Source: CAD feature listing. Evaluate the final solid. Frame: model axes, mm. A direction names the side the tool comes from. Give positions to 0.01 mm unless a question says otherwise; leave off trailing zeros. Order: outer loops, then holes, each group sorted by start corner. A loop starts at its lowest first (then second) coordinate and runs counter-clockwise, first axis right, second up.
1) First-contact query: P1, Ø8.5, axis at y = 16, z = -265.5, coming from the +X side; P2, Ø3, axis at x = -2, z = -152.5, coming from the +Y side; P3, Ø4, axis at y = 10, z = -219, coming from the -X side. Flat tips, straight axial feed; report the tip coordinate or a pass-through.
2) Access query for faces 1 (the face through (-9, 25, 0)), 2 (the face through (-5.622, 33, -211)), 3 (the face through (-9, 25, -428.625)), 4 (the face through (-6.511, 32, -211)), 5 (the face through (-2.967, 3.174, -211.312)). Directions: +Z, -Z, +X, -X, +Y, -Y. A direction counts if a zero-diameter tool reaches every point of the face in a straight line with its end or side. Return the directions, or none.
3) Draft query along Y for faces 6 (the face through (-10.739, 42.804, -211.312)), 7 (the face through (-8.767, 16, -211)), 8 (the face through (-3.45, 2.413, -211.312)), 9 (the face through (-9.656, 16, -211)). Return one class per face: released by +Y, released by -Y, zero draft, split by the parting line, or undercut.
4) Section A-A, the plane x = -2.25. Return loops of the section in (y, z) (3 decimals), plus the area to 3 significant figures.
5) Section C-C, the plane y = 15. Return loops of the section in (x, z) (3 decimals), plus the area to 3 significant figures.
6) Material intervals for line 1 (X direction, y = 32.5, z = -94); line 2 (X direction, y = 29, z = -211.5); line 3 (X direction, y = 20, z = -220.5), sorted ascending.
```python
from build123d import *

# Parameters (mm, degrees)
EXTRUDE_THIN1_DEPTH = 428.625
FILLET1_R           = 0.889


with BuildPart() as part:
    # Sketch1 → Extrude-Thin1 (new body)
    with BuildSketch(Plane.XY):
        with BuildLine():
            ThreePointArc((0, 0), (4.964730566, 2.465229927), (7.9375, 7.14375))
            Line((7.9375, 7.14375), (11.1125, 7.14375))
            Line((11.1125, 7.14375), (11.1125, 24.60625))
            ThreePointArc((11.1125, 24.60625), (12.04243597, 26.85131403), (14.2875, 27.78125))
            Line((14.2875, 27.78125), (13.517722525, 32.146875))
            Line((13.517722525, 32.146875), (16.898645987, 34.098852071))
            ThreePointArc((16.898645987, 34.098852071), (18.624416275, 36.126706761), (18.680023291, 38.788921177))
            ThreePointArc((18.680023291, 38.788921177), (12.079369103, 42.78588283), (7.078269835, 36.909375))
            Line((7.078269835, 36.909375), (7.078269835, 28.178125))
            Line((7.078269835, 28.178125), (0.728269835, 28.178125))
            Line((0.728269835, 28.178125), (0.728269835, 27.289125))
            Line((0.728269835, 27.289125), (7.967269835, 27.289125))
            Line((7.967269835, 27.289125), (7.967269835, 36.909375))
            ThreePointArc((7.967269835, 36.909375), (12.221538279, 41.908324327), (17.836494775, 38.508242281))
            ThreePointArc((17.836494775, 38.508242281), (17.79334373, 36.442363895), (16.454145987, 34.868748655))
            Line((16.454145987, 34.868748655), (12.534135133, 32.605529333))
            Line((12.534135133, 32.605529333), (13.251696834, 28.536034702))
            ThreePointArc((13.251696834, 28.536034702), (11.068369678, 27.086833796), (10.2235, 24.60625))
            Line((10.2235, 24.60625), (10.2235, 8.03275))
            Line((10.2235, 8.03275), (7.254256557, 8.03275))
            ThreePointArc((7.254256557, 8.03275), (4.608977552, 3.348689722), (-0.166979013, 0.873177536))
            Line((-0.166979013, 0.873177536), (0, 0))
        make_face()
    extrude(amount=-EXTRUDE_THIN1_DEPTH)

    # Fillet1
    fillet1_edges = [part.edges().sort_by_distance(p)[0] for p in [
        (14.2875, 27.78125, -214.3125),
        (11.1125, 7.14375, -214.3125),
        (7.254256557, 8.03275, -214.3125),
        (12.534135133, 32.605529333, -214.3125),
        (7.967269835, 27.289125, -214.3125),
    ]]
    fillet(fillet1_edges, radius=FILLET1_R)


with BuildPart() as body_2:
    # Mirror1: mirrored copy
    add(part.part.mirror(Plane(origin=(0.728269835, 27.289125, -428.625), x_dir=(0, 0, 1), z_dir=(1, 0, 0))))


solid = body_2.part
```
From the geometry:
1. P1: stops at x = -8.77
1. P2: stops at y = 28.18
1. P3: stops at x = -9.66
2. face 1: +Z, +X, -X, +Y, -Y
2. face 2: +Z, -Z, +X, +Y
2. face 3: -Z, +X, -X, +Y, -Y
2. face 4: +Z, -Z
2. face 5: +Z, -Z, +X
3. face 6: released by +Y
3. face 7: undercut
3. face 8: released by -Y
3. face 9: zero draft
4. outline: (1.497, -428.625) - (2.581, -428.625) - (2.581, 0) - (1.497, 0) - close; (27.289, -428.625) - (28.178, -428.625) - (28.178, 0) - (27.289, 0) - close
4. area: 846 mm2
5. outline: (-9.656, -428.625) - (-8.767, -428.625) - (-8.767, 0) - (-9.656, 0) - close
5. area: 381 mm2
6. line 1: x = -12.67 to -11.25, -6.51 to -5.62
6. line 2: x = -12.62 to -11.71, -6.51 to -5.62
6. line 3: x = -9.66 to -8.77
